```python
from build123d import *

# Parameters (mm, degrees)
BOSS_EXTRUDE1_DEPTH = 25.4
FILLET1_R           = 12.7
FILLET2_R           = 7.62
CUT_EXTRUDE1_DEPTH  = 21.59
SKETCH3_R           = 4.7625
CUT_EXTRUDE2_DEPTH  = 2.54
SKETCH4_R           = 2.38125
CUT_EXTRUDE3_DEPTH  = 58.938313101


with BuildPart() as part:
    # Sketch1 → Boss-Extrude1 (new body)
    with BuildSketch(Plane.XY):
        with BuildLine():
            ThreePointArc((-28.575, 0), (0, 28.575), (28.575, 0))
            Line((28.575, 0), (28.575, -25.4))
            Line((28.575, -25.4), (41.275, -25.4))
            Line((41.275, -25.4), (41.275, 0))
            Line((41.275, 0), (31.75, 0))
            ThreePointArc((31.75, 0), (0, 31.75), (-31.75, 0))
            Line((-31.75, 0), (-28.575, 0))
        make_face()
    extrude(amount=BOSS_EXTRUDE1_DEPTH)

    # Fillet1
    # the kernel refuses this fillet: 12.7 mm, written as the material it adds along each edge
    with BuildSketch(Plane(origin=(31.75, 0, 0), x_dir=(1, 0, 0), z_dir=(0, 0, 1))) as fillet1_piece_1:
        with BuildLine():
            CenterArc((10.868269231, 12.628761926), FILLET1_R, 196.505753727, 67.422759238)
            Line((-1.308379121, 9.020544233), (-1.551912088, 8.948379879))
            ThreePointArc((-1.551912088, 8.948379879), (-0.580166885, 4.521008688), (-0.254, 0))
            Line((-0.254, 0), (0, -0.254))
            ThreePointArc((0, -0.254), (4.7625, -0.254), (9.498134615, -0.252575239))
            Line((9.498134615, -0.252575239), (9.525, 0))
        make_face()
    extrude(amount=25.4)

    # Fillet2
    fillet2_edges = [part.edges().sort_by_distance(p)[0] for p in [
        (41.275, 0, 12.7),
    ]]
    fillet(fillet2_edges, radius=FILLET2_R)

    # Sketch2 → Cut-Extrude1 (cut)
    with BuildSketch(Plane(origin=(0, -25.4, 0), x_dir=(-1, 0, 0), z_dir=(0, -1, 0))):
        with BuildLine():
            ThreePointArc((-38.474757914, -9.525), (-39.6875, -12.7), (-38.474757914, -15.875))
            Line((-38.474757914, -15.875), (-31.375242086, -15.875))
            ThreePointArc((-31.375242086, -15.875), (-30.47600414, -14.399365203), (-30.1625, -12.7))
            ThreePointArc((-30.1625, -12.7), (-30.47600414, -11.000634797), (-31.375242086, -9.525))
            Line((-31.375242086, -9.525), (-38.474757914, -9.525))
        make_face()
    extrude(amount=-CUT_EXTRUDE1_DEPTH, mode=Mode.SUBTRACT)

    # Sketch3 → Cut-Extrude2 (cut)
    with BuildSketch(Plane.XZ.offset(25.4)):
        with Locations(Location((34.925, 12.7, 0), (0, 0, 270))):
            Circle(SKETCH3_R)
    extrude(amount=-CUT_EXTRUDE2_DEPTH, mode=Mode.SUBTRACT)

    # Sketch4 → Cut-Extrude3 (cut, through all)
    with BuildSketch(Plane.XY.offset(25.4)):
        with Locations((34.925, -20.32)):
            Circle(SKETCH4_R)
    extrude(amount=-CUT_EXTRUDE3_DEPTH, mode=Mode.SUBTRACT)


solid = part.part
```
Input: part model. Units: mm. Frame: model coordinates. A direction names the side the tool comes from. Coordinates: 2 decimals unless noted, no trailing zeros. Write each loop counter-clockwise with the first axis right and the second up, starting at its lowest first coordinate (ties: lowest second). Pieces come first, ordered by that corner, then holes. Notation, with made-up numbers: (-9, 76.5) -> (38, 76.5) arc R20 ccw to (38, 92.5) -> close; hole circle Ø5 at (81, 81). An arc over 180 degrees is marked (long way). Write each question's results on one line, items separated by ' | '.
Item 1: Section query B-B on y = -20.32. Return loops of the section in (x, z) (1 decimal).
Conclusion:
outline: (28.6, 0) -> (32.5, 0) -> (32.5, 9.5) -> (31.4, 9.5) arc R4.8 cw to (31.4, 15.9) -> (32.5, 15.9) -> (32.5, 25.4) -> (28.6, 25.4) -> close; (37.3, 0) -> (41.3, 0) -> (41.3, 25.4) -> (37.3, 25.4) -> (37.3, 15.9) -> (38.5, 15.9) arc R4.8 cw to (38.5, 9.5) -> (37.3, 9.5) -> close
Item 2: Pin query (flat end, axial travel): pin 1 Ø2.5 at (x, z) = (-30.5, 14) entering from -Y; pin 2 Ø10 at (x, z) = (17.5, 15.5) entering from +Y; pin 3 Ø0.8 at (x, z) = (35.5, 8.5) entering from -Y. Return the tip coordinate at first contact, or that it passes through.
Conclusion:
pin 1: stops at y = 0 | pin 2: stops at y = 29.19 | pin 3: stops at y = -22.86
Item 3: Section query C-C on y = -14. Return loops of the section in (x, z) (1 decimal), plus the area to 3 significant figures.
Conclusion:
outline: (28.6, 0) -> (41.3, 0) -> (41.3, 25.4) -> (28.6, 25.4) -> close; hole (31.4, 9.5) -> (38.5, 9.5) arc R4.8 ccw to (38.5, 15.9) -> (31.4, 15.9) arc R4.8 ccw to start | area: 267 mm^2
Item 4: Material intervals for probe 1 along X at (y, z) = (-20, 13) (3 decimals); probe 2 along X at (y, z) = (-16, 15) (3 decimals); probe 3 along X at (y, z) = (-13, 22.25) (3 decimals), sorted ascending.
Conclusion:
probe 1: x = 28.575 to 30.172, 39.678 to 41.275 | probe 2: x = 28.575 to 30.755, 39.095 to 41.275 | probe 3: x = 28.575 to 41.275
Item 5: Set-up query: faces 5 (the flat face through (28.575, -13, 13)), 6 (the flat face through (35, -22.86, 9)), 7 (the flat face through (39.1, -25.4, 9.7)). Return all of +Z, -Z, +X, -X, +Y, -Y with unobstructed straight access to the full face (end or side cutting, diameter ignored); none if empty.
Conclusion:
face 5: +Z, -Z, -X, -Y | face 6: -Y | face 7: +Z, -Z, +X, -X, -Y
Item 6: Mould query, pull axis Z, two halves, no side actions, for faces 1 (the flat face through (29, 3, 0)), 2 (the flat face through (-30, 0, 13)), 3 (the flat face through (35, -11, 15.875)), 4 (the flat face through (29, 3, 25.4)). Classes: +Z half, -Z half, draft (parallel to the pull), parting line (faces both ways), or undercut.
Conclusion:
face 1: -Z half | face 2: draft | face 3: undercut | face 4: +Z half
Item 7: Section query D-D on x = 0. Return loops of the section in (y, z) (3 decimals), plus the area to 3 significant figures.
Conclusion:
outline: (28.575, 0) -> (31.75, 0) -> (31.75, 25.4) -> (28.575, 25.4) -> close | area: 80.6 mm^2
